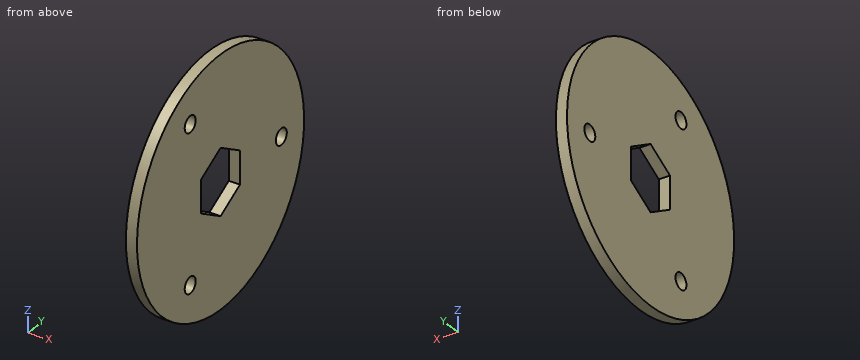
```python
from build123d import *

# Parameters (mm, degrees)
SKETCH1_R           = 27.5
SKETCH1_R_2         = 1.8
BOSS_EXTRUDE1_DEPTH = 2.5


with BuildPart() as part:
    # Sketch1 → Boss-Extrude1 (new body)
    with BuildSketch(Plane(origin=(0, 0, 0), x_dir=(0, 0, -1), z_dir=(1, 0, 0))):
        Circle(SKETCH1_R)
        with Locations((0, 20)):
            Circle(SKETCH1_R_2, mode=Mode.SUBTRACT)
        with Locations((-17.320508076, -10)):
            Circle(SKETCH1_R_2, mode=Mode.SUBTRACT)
        with Locations((17.320508076, -10)):
            Circle(SKETCH1_R_2, mode=Mode.SUBTRACT)
        Polygon((3.680607966, 6.375), (-3.680607966, 6.375), (-7.361215932, 0), (-3.680607966, -6.375), (3.680607966, -6.375), (7.361215932, 0), align=None, mode=Mode.SUBTRACT)
    extrude(amount=BOSS_EXTRUDE1_DEPTH)


solid = part.part
```
The listing builds one solid part. Answer for the finished solid, in the listing's coordinates (mm). Give positions to 0.01 mm unless a question says otherwise; leave off trailing zeros. Loops run counter-clockwise (first coordinate to the right, second up) from the corner with the lowest first, then second, coordinate; pieces in that order, holes last. Notation, with made-up numbers: (-19.75, 70) - (7.25, 70) arc R33 ccw to (7.25, 107) - close; hole circle Ø5 at (-34, 88). An arc over 180 degrees is marked (long way). Return JSON: item names as keys, results as strings. Group by question number.
1. Find section C-C (x = 1.75). Write down the section's boundary in (y, z) (1 decimal).
2. Find section D-D (y = -9). Write down the section's boundary in (x, z).
3. Straight lines are drawn through the part: line 1 (Y direction, x = 0.85, z = 0) (3 decimals); line 2 (Z direction, x = 1.65, y = -9.5); line 3 (Z direction, x = 1.35, y = -1). For each, find the intervals that lie inside material, in ascending order. Write a range as [from, to].
4. Given pin 1 Ø1.5 at (x, z) = (1, -0.5) entering from +Y; pin 2 Ø1.5 at (x, z) = (0.5, 12) entering from +Y; pin 3 Ø3 at (y, z) = (-10, -17.32) entering from -X; pin 4 Ø4.5 at (y, z) = (-10, 17.32) entering from -X, each flat-ended and moving along its own axis, determine where each tip first touches the part or whether it passes through.
5. Find section A-A (z = 0). Write down the section's boundary in (x, y) (3 decimals).
6. Find section B-B (y = 20). Write down the section's boundary in (x, z).
Verdict:
{
 "1": {"outline": "circle Ø55 at (0, 0); hole circle Ø3.6 at (-10, -17.3); hole circle Ø3.6 at (-10, 17.3); hole (-6.4, -3.7) - (0, -7.4) - (6.4, -3.7) - (6.4, 3.7) - (0, 7.4) - (-6.4, 3.7) - close; hole circle Ø3.6 at (20, 0)"},
 "2": {"outline": "(0, -25.99) - (2.5, -25.99) - (2.5, -18.82) - (0, -18.82) - close; (0, -15.82) - (2.5, -15.82) - (2.5, 15.82) - (0, 15.82) - close; (0, 18.82) - (2.5, 18.82) - (2.5, 25.99) - (0, 25.99) - close"},
 "3": {"line 1": "y = [-27.5, -6.375], [6.375, 18.2], [21.8, 27.5]", "line 2": "z = [-25.81, -19.05], [-15.59, 15.59], [19.05, 25.81]", "line 3": "z = [-27.48, -6.78], [6.78, 27.48]"},
 "4": {"pin 1": "stops at y = 27.5", "pin 2": "stops at y = 25.09", "pin 3": "passes through", "pin 4": "stops at x = 0"},
 "5": {"outline": "(0, -27.5) - (2.5, -27.5) - (2.5, -6.375) - (0, -6.375) - close; (0, 6.375) - (2.5, 6.375) - (2.5, 18.2) - (0, 18.2) - close; (0, 21.8) - (2.5, 21.8) - (2.5, 27.5) - (0, 27.5) - close"},
 "6": {"outline": "(0, -18.87) - (2.5, -18.87) - (2.5, -1.8) - (0, -1.8) - close; (0, 1.8) - (2.5, 1.8) - (2.5, 18.87) - (0, 18.87) - close"}
}
